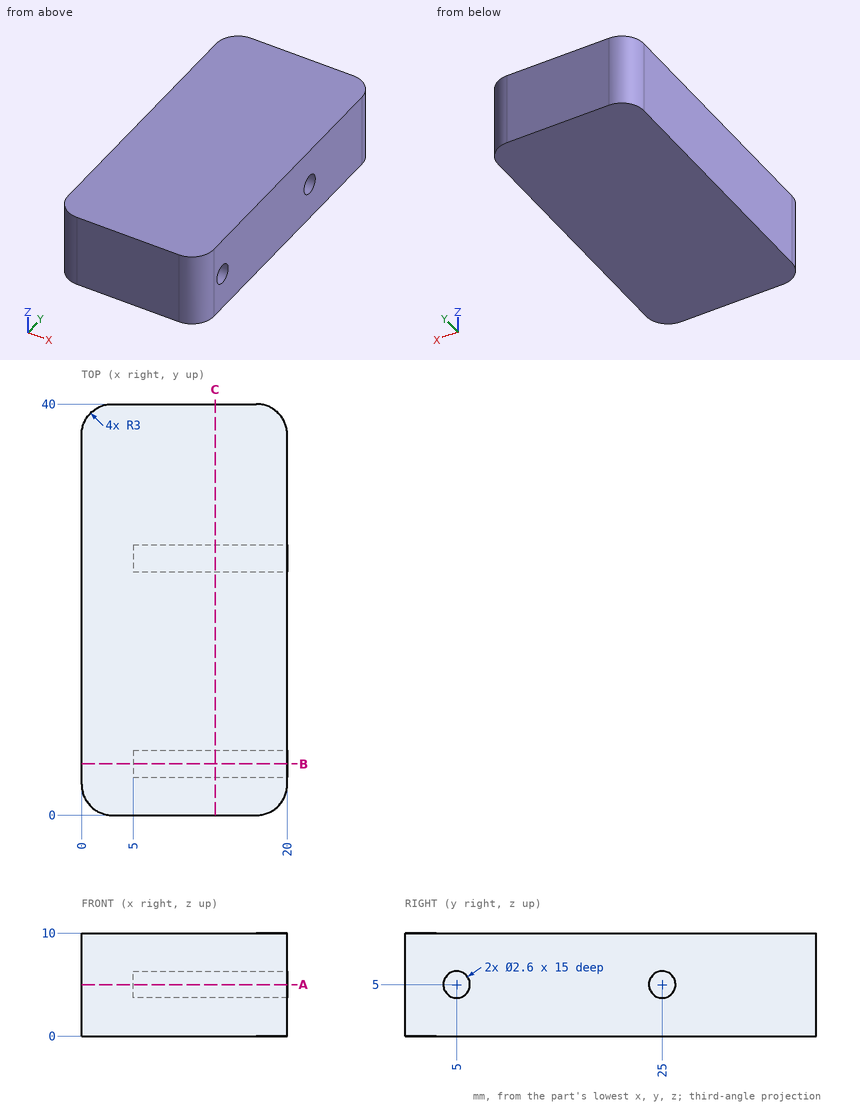
Print and shaded views of the part. All mm, measured from the part's lowest x, y and z. Coordinates: 2 decimals unless noted, no trailing zeros. Write each loop counter-clockwise with the first axis right and the second up, starting at its lowest first coordinate (ties: lowest second). Pieces come first, ordered by that corner, then holes. Notation, with made-up numbers: (69, 82.25) - (124, 82.25) arc R12 ccw to (124, 88.25) - close; hole circle Ø1 at (-35.75, 84.25). An arc over 180 degrees is marked (long way). One line per question, with ' | ' between items. Start each with the question number.
Q1. Cut at B-B, the plane y = 5. List the corners of the cut face in (x, z).
Q2. Drill centre lines: line 1 (Y direction, x = 8, z = 5); line 2 (Z direction, x = 16, y = 24.5); line 3 (Y direction, x = 18.75, z = 8.5). Where is each one in solid material? Low to high. Write a range as [from, to].
Q3. Cut at A-A, the plane z = 5. List the corners of the cut face in (x, y), then the cut area to 3 significant figures.
Q4. Cut at C-C, the plane x = 13. List the corners of the cut face in (y, z).
Q5. Pin check, flat tips, straight feed: pin 1 (6 mm diameter, centred on x = 16, z = 7, fed in from -Y); pin 2 (1.3 mm diameter, centred on y = 5, z = 5, fed in from +X). Stop position of each tip, or through.
Answer below:
1) outline: (0, 0) - (20, 0) - (20, 3.7) - (5, 3.7) - (5, 6.3) - (20, 6.3) - (20, 10) - (0, 10) - close
2) line 1: [0, 3.7], [6.3, 23.7], [26.3, 40] | line 2: [0, 3.8], [6.2, 10] | line 3: [0.56, 39.44]
3) outline: (0, 3) arc R3 ccw to (3, 0) - (17, 0) arc R3 ccw to (20, 3) - (20, 3.7) - (5, 3.7) - (5, 6.3) - (20, 6.3) - (20, 23.7) - (5, 23.7) - (5, 26.3) - (20, 26.3) - (20, 37) arc R3 ccw to (17, 40) - (3, 40) arc R3 ccw to (0, 37) - close | area: 714 mm^2
4) outline: (0, 0) - (40, 0) - (40, 10) - (0, 10) - close; hole circle Ø2.6 at (5, 5); hole circle Ø2.6 at (25, 5)
5) pin 1: y = 0 | pin 2: x = 5
